Check sheet for the drawn part. Datum: minimum x, y, z corner. Units: mm. A direction names the side the tool comes from. Round coordinates to 2 decimals unless told otherwise and drop trailing zeros. Loops run counter-clockwise (first coordinate to the right, second up) from the corner with the lowest first, then second, coordinate; pieces in that order, holes last.
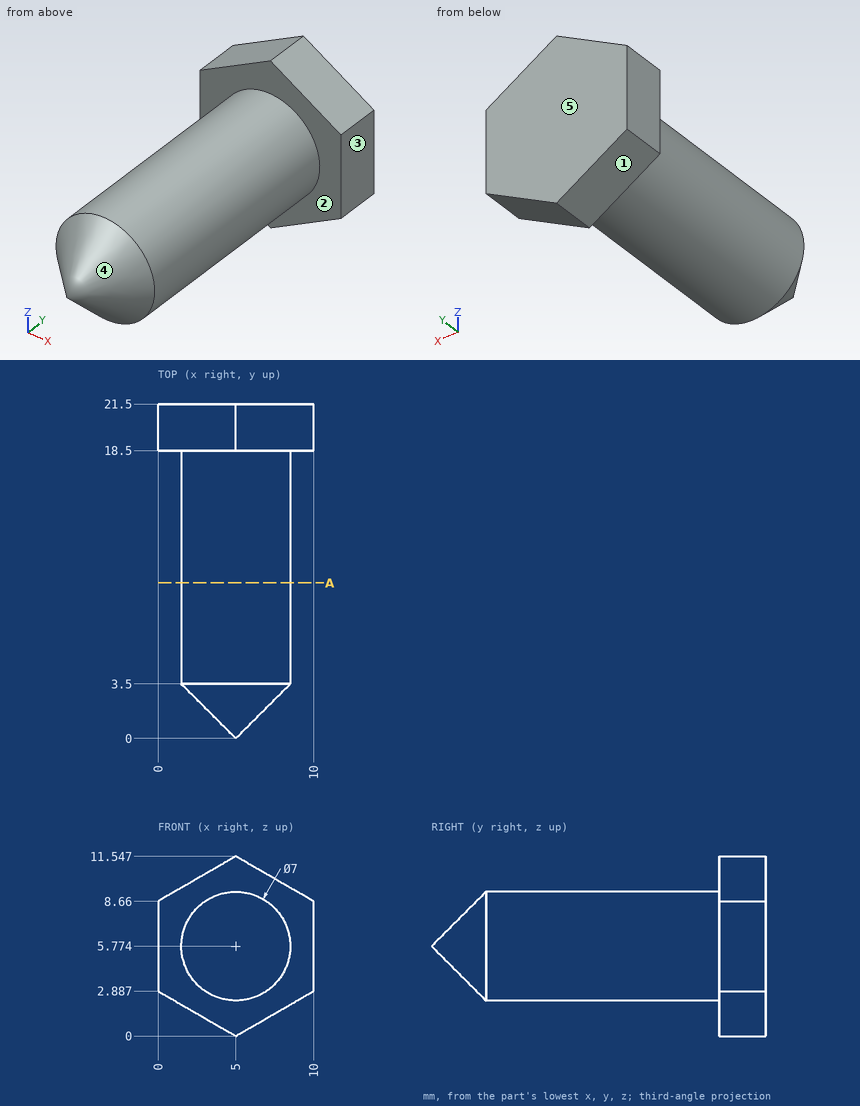
1. Tool access check on the marked faces 1 and 2. Record the directions out of +Z, -Z, +X, -X, +Y, -Y that give a thin tool (end or side, any length) a straight path to the whole face; none if there is none.
2. Gauge pin test, flat ends, axial feed: P1, Ø5, axis at y = 3.5, z = 4, coming from the +X side; P2, Ø5, axis at x = 7.5, y = 4, coming from the +Z side; P3, Ø5, axis at x = 8, z = 2.5, coming from the -Y side. Record the tip position at first contact, or that the pin passes through.
3. Release check for a two-part mould opening along Y. For the marked faces 3, 4 and 5 record: released by +Y, released by -Y, zero draft, split by the parting line, or undercut.
4. Section check A-A (y = 10). Enter the section's corners in (x, z), then the cut area to 3 significant figures.
5. Scan lines: L1, parallel to X at y = 6.75, z = 5.75; L2, parallel to Y at x = 3.5, z = 2.5; L3, parallel to X at y = 9.5, z = 3.75 (1 decimal). Record each from-to range of solid material in increasing order.
Taken from the geometry:
1. face 1: -Z, -X, +Y, -Y
1. face 2: -Y
2. P1: stops at x = 8.5
2. P2: stops at z = 9.27
2. P3: stops at y = 1.94
3. face 3: zero draft
3. face 4: released by -Y
3. face 5: released by +Y
4. outline: circle Ø7 at (5, 5.77)
4. area: 38.5 mm2
5. L1: x = 1.5 to 8.5
5. L2: y = 18.5 to 21.5
5. L3: x = 2.1 to 7.9
